Read the model definition and answer for the solid it produces. Units are mm, in the model's axes. A direction names the side the tool comes from. Coordinates: 2 decimals unless noted, no trailing zeros. Write each loop counter-clockwise with the first axis right and the second up, starting at its lowest first coordinate (ties: lowest second). Pieces come first, ordered by that corner, then holes.
Item 1: Section A-A (x = 14.5) is taken. Give the vertices of the cut face in (y, z), then the cut area to 3 significant figures.
Item 2: Each of these flat-tipped pins is pushed along its axis until it touches: P1, Ø3.5, axis at y = 0, z = 0, coming from the -X side; P2, Ø1, axis at x = 0, y = 0, coming from the +Z side; P3, Ø0.5, axis at y = 0.5, z = 0, coming from the -X side; P4, Ø1, axis at x = -19, y = 1.5, coming from the -Z side. Where does it stop, or does it pass through?
Item 3: Section C-C (y = -0.5) is taken. State how many separate pieces and enclosed holes the cut face has, then the cut area to 3 significant figures.
Item 4: Straight lines are drawn through the part: probe 1 along X at (y, z) = (0, -3.05); probe 2 along Y at (x, z) = (6, 0). For each, find the intervals that lie inside material, in ascending order.
Item 5: A tool of negligible diameter and unlimited length cuts with its end or side. For faces 4 (the face through (-19, 0, 0.75)), 5 (the face through (-20, 0, 2)), from which of +Z, -Z, +X, -X, +Y, -Y can it reach the whole face along a straight path? Write none if from no direction.
Item 6: Determine the mould class of faces 1 (the face through (-19.86, -0.07, -3.64)), 2 (the face through (0.785, -0.326, -2.681)), 3 (the face through (9.353, -0.091, 2.065)) for opening direction Z: released by +Z, released by -Z, zero draft, split by the parting line, or undercut.
Item 7: Section B-B (x = -3) is taken. Give the vertices of the cut face in (y, z).
Autodesk Inventor part; units mm, degrees
ref_plane "YZ Plane" through (0, 0, 0) normal (1, 0, 0) x (0, 1, 0)
ref_plane "XZ Plane" through (0, 0, 0) normal (0, 1, 0) x (-1, 0, 0)
ref_plane "XY Plane" through (0, 0, 0) normal (0, 0, 1) x (1, 0, 0)
sketch "Skizze1" plane through (0, 0, 0) normal (0, 0, 1) x (1, 0, 0)
  line L0 (0, 0) -> (24.9383, 0)
  line L1 (20, 0) -> (-20, 0)
  line L2 (-20, 0) -> (-20, 4)
  line L3 (-20, 4) -> (20, 4)
  line L4 (20, 4) -> (20, 0)
  circle A0 centre (0, 0) radius 0.85
  dimension "d0" = 40
  dimension "d1" = 8
  dimension "d2" = 1.7
revolve "Umdrehung1" add sketch "Skizze1" angle 360 about axis through (0, 0, 0) along (1, 0, 0) picked at (-0.5584, 0.0678) contours L1 A0 L0 | A0 L1 L2 L3 L4 L0
sketch "Skizze2" plane through (0, 0, 0) normal (0, 0, 1) x (1, 0, 0)
  circle A0 centre (0, 0) radius 0.85
extrude "Extrusion1" cut sketch "Skizze2" along normal through all both and the other way through all
sketch "Skizze3" plane through (20, 0, 0) normal (1, 0, 0) x (0, 0, -1)
  point P0 (0, 0)
  point P1 (0, 0)
hole "Bohrung1" at (20, 0, 0) direction (-1, 0, 0) diameter 4.134 depth 21 tip angle 118
chamfer "Fase1" distance 0.5 angle 45 2 edges at (20, -4, 0) (-20, -4, 0)
chamfer "Fase2" distance 0.5 angle 45 2 edges at (-0.85, -0.0027, -4) (-0.85, -0.0027, 4)
sketch "Sketch4" plane through (-20, 0, 0) normal (-1, 0, 0) x (0, 0, 1)
  line L0 (0.75, -4) -> (-0.75, -4)
  line L1 (-0.75, -4) -> (-0.75, 4)
  line L2 (-0.75, 4) -> (0.75, 4)
  line L3 (0.75, 4) -> (0.75, -4)
  line L4 (0.75, -4) -> (-0.75, 4) construction
  line L5 (-0.75, -4) -> (0.75, 4) construction
  circle A0 centre (0, 0) radius 4
  point P0 (0.75, 3.9291)
  point P1 (-0.75, 3.9291)
  point P2 (-0.75, -3.9291)
  point P3 (0.75, -3.9291)
  dimension "d19" = 1.5
extrude "Extrusion2" cut sketch "Sketch4" against normal blind 2 contours A0 L1 L3
properties part number "bolt_V1" material "Stahl, Legierung"
Established:
1. outline: circle Ø8 at (0, 0); hole circle Ø4.13 at (0, 0)
1. area: 36.8 mm2
2. P1: stops at x = -20
2. P2: passes through
2. P3: stops at x = -18
2. P4: stops at z = -3.87
3. separate pieces: 3
3. enclosed holes: 0
3. area: 222 mm2
4. probe 1: x = -20 to -0.85, 0.85 to 20
4. probe 2: y = -4 to -2.07, 2.07 to 4
5. face 4: -X, +Y, -Y
5. face 5: +Z, -Z, -X, +Y, -Y
6. face 1: released by -Z
6. face 2: zero draft
6. face 3: undercut
7. outline: circle Ø8 at (0, 0)
